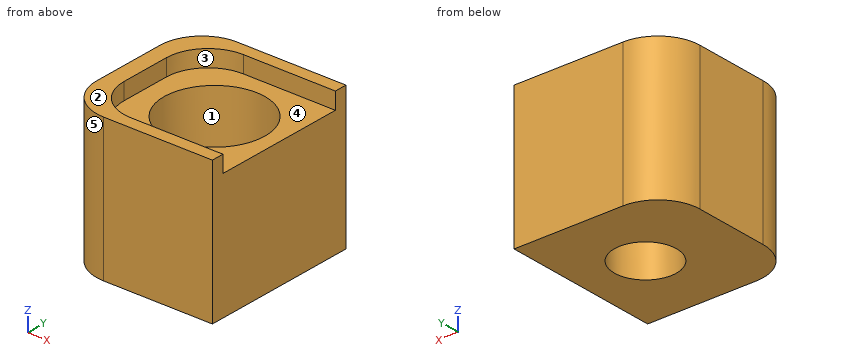
from build123d import *

# Parameters (mm, degrees)
F0_W          = 16
F0_H          = 16
F0_R          = 6
F0_R_2        = 3.7
F1_DEPTH      = 15
F2_DEPTH      = 2
F2_DEPTH_BACK = 15
F3_R          = 5
F4_DEPTH      = 10


with BuildPart() as f1:
    # F0 (on Top) → F1 (new body)
    with BuildSketch(Plane.XY):
        Rectangle(F0_W, F0_H)
        with Locations((0.285, 0)):
            Circle(F0_R, mode=Mode.SUBTRACT)
        with Locations((0.285, 0)):
            Circle(F0_R)
        with Locations((0.285, 0)):
            Circle(F0_R_2, mode=Mode.SUBTRACT)
    extrude(amount=-F1_DEPTH)

    # F0 (on Top) → F2 (join, two sides)
    with BuildSketch(Plane.XY) as f2_sk:
        Polygon((8, -9.5), (8, -8), (-8, -8), (-8, 8), (8, 8), (8, 9.5), (-10, 9.5), (-10, -9.5), align=None)
    extrude(amount=F2_DEPTH)
    extrude(f2_sk.sketch, amount=-F2_DEPTH_BACK)

    # F3
    f3_edges = [f1.edges().sort_by_distance(p)[0] for p in [
        (-8, 8, 1),
        (-8, -8, 1),
        (-10, 9.5, -6.5),
        (-10, -9.5, -6.5),
    ]]
    fillet(f3_edges, radius=F3_R)

    # F0 (on Top) → F4 (cut)
    with BuildSketch(Plane.XY):
        with Locations((0.285, 0)):
            Circle(F0_R)
        with Locations((0.285, 0)):
            Circle(F0_R_2, mode=Mode.SUBTRACT)
    extrude(amount=-F4_DEPTH, mode=Mode.SUBTRACT)


solid = f1.part
Here's how the part is built. I have some questions about the finished solid (model axes, mm). Face numbers are marked on the shaded views. A direction names the side the tool comes from. Round coordinates to 2 decimals unless told otherwise and drop trailing zeros. Order: outer loops, then holes, each group sorted by start corner. A loop starts at its lowest first (then second) coordinate and runs counter-clockwise, first axis right, second up. Notation, with made-up numbers: M 50.5,19 L 67.5,19 A20 ccw 67.5,40 Z; hole C 89,51.5 d11. An arc over 180 degrees is marked long. Return JSON: item names as keys, results as strings. Group by question number.
1. Please list where these lines run through material, in increasing order: probe 1 along Y at (x, z) = (0.25, -13.5); probe 2 along Y at (x, z) = (5.5, 0.75); probe 3 along Z at (x, y) = (2.5, 5).
2. If we mould it in two halves opening along X, with no side actions, what happens to the marked faces 1, 2 and 3? For each: pulls with the +X half, pulls with the -X half, needs draft (parallel to the pull), parting line crosses it, or undercut.
3. If we section it at B-B on z = -5.75: List the corners of the cut face in (x, y) for me (3 decimals), then the cut area to 3 significant figures.
4. If we section it at C-C on x = 1.5: List the corners of the cut face in (y, z) for me, then the cut area to 3 significant figures.
5. I'm going to push flat-ended pins straight in: pin 1 Ø5 at (x, y) = (4, 2) entering from +Z; pin 2 Ø2 at (y, z) = (-0.5, 1.5) entering from +X. Where does each tip first touch, or does it pass through?
6. On a 3-axis mill with a long thin cutter (end or side, diameter ignored), from which of +Z, -Z, +X, -X, +Y, -Y can I reach the whole of each face in a straight line? I mean the marked faces 4 and 5. Say none if no direction works.
7. If we section it at A-A on y = 0: List the corners of the cut face in (x, z) for me (3 decimals), then the cut area to 3 significant figures.
8. If we section it at D-D on x = -3.75: List the corners of the cut face in (y, z) for me, then the cut area to 3 significant figures.
Reply:
{
 "1": {"probe 1": "-9.5 to -3.7, 3.7 to 9.5", "probe 2": "-9.5 to -8, 8 to 9.5", "probe 3": "-15 to -10"},
 "2": {"face 1": "undercut", "face 2": "needs draft", "face 3": "pulls with the +X half"},
 "3": {"outline": "M -10,-4.5 A5 ccw -5,-9.5 L 8,-9.5 L 8,9.5 L -5,9.5 A5 ccw -10,4.5 Z; hole C 0.285,0 d12", "area": "218 mm^2"},
 "4": {"outline": "M -9.5,-15 L -3.49,-15 L -3.49,-10 L -5.88,-10 L -5.88,0 L -8,0 L -8,2 L -9.5,2 Z; M 3.49,-15 L 9.5,-15 L 9.5,2 L 8,2 L 8,0 L 5.88,0 L 5.88,-10 L 3.49,-10 Z", "area": "139 mm^2"},
 "5": {"pin 1": "z = 0", "pin 2": "x = -8"},
 "6": {"face 4": "+Z, +X", "face 5": "+Z, -Z, -X, -Y"},
 "7": {"outline": "M -10,-15 L -3.415,-15 L -3.415,-10 L -5.715,-10 L -5.715,0 L -8,0 L -8,2 L -10,2 Z; M 3.985,-15 L 8,-15 L 8,0 L 6.285,0 L 6.285,-10 L 3.985,-10 Z", "area": "117 mm^2"},
 "8": {"outline": "M -9.5,-15 L 9.5,-15 L 9.5,2 L 7.94,2 L 7.94,0 L 4.44,0 L 4.44,-10 L -4.44,-10 L -4.44,0 L -7.94,0 L -7.94,2 L -9.5,2 Z", "area": "202 mm^2"}
}
